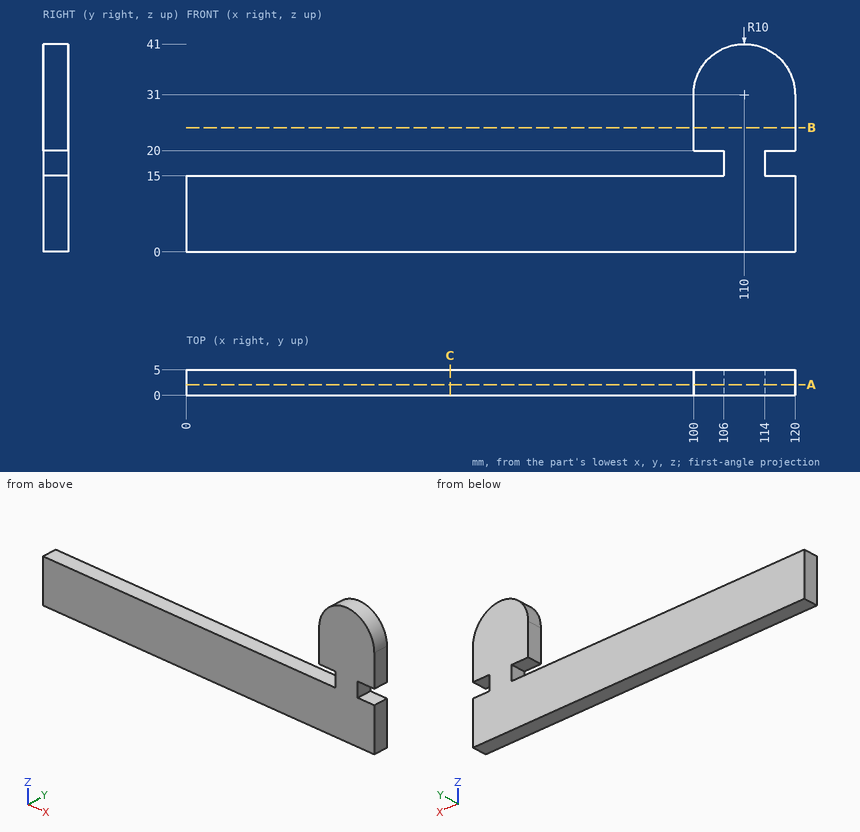
Could you check a few things on this drawing? It's one solid part, dimensions in mm from its lowest x, y, z. Round coordinates to 2 decimals unless told otherwise and drop trailing zeros. Loops run counter-clockwise (first coordinate to the right, second up) from the corner with the lowest first, then second, coordinate; pieces in that order, holes last. Notation, with made-up numbers: M 26.5,82 L 53.5,82 A16 ccw 53.5,86 Z; hole C 17.25,29.25 d4. An arc over 180 degrees is marked long. Write each question's results on one line, items separated by ' | '. Start each with the question number.
(1) Will these pins go through, and if not, where does the flat tip stop? P1, Ø2.5, axis at y = 3, z = 17.5, coming from the +X side; P2, Ø1.5, axis at y = 1.5, z = 17.5, coming from the -X side.
(2) If I drill on probe 1 along X at (y, z) = (0.65, 28); probe 2 along X at (y, z) = (2.1, 16.5); probe 3 along Z at (x, y) = (76.5, 0.95), over which ranges is the centre line in solid material (lowest first)? Write a range as from..to.
(3) I want a section at A-A (y = 2.1). Please give me the cut outline in (x, z), then the cut area to 3 significant figures.
(4) I want a section at B-B (z = 24.5). Please give me the cut outline in (x, y), then the cut area to 3 significant figures.
(5) I want a section at C-C (x = 52). Please give me the cut outline in (y, z).
Solved:
1) P1: stops at x = 114 | P2: stops at x = 106
2) probe 1: x = 100..120 | probe 2: x = 106..114 | probe 3: z = 0..15
3) outline: M 0,0 L 120,0 L 120,15 L 114,15 L 114,20 L 120,20 L 120,31 A10 ccw 100,31 L 100,20 L 106,20 L 106,15 L 0,15 Z | area: 2,220 mm²
4) outline: M 100,0 L 120,0 L 120,5 L 100,5 Z | area: 100 mm²
5) outline: M 0,0 L 5,0 L 5,15 L 0,15 Z
